Design review of the part shown in the three views and the two pictorial views. Dimensions are in mm from the part's minimum x, y and z. Give positions to 0.01 mm unless a question says otherwise; leave off trailing zeros. Loops run counter-clockwise (first coordinate to the right, second up) from the corner with the lowest first, then second, coordinate; pieces in that order, holes last. Notation, with made-up numbers: (64, 32) -> (93, 32) arc R20 ccw to (93, 54) -> close; hole circle Ø10 at (26, 57.25). An arc over 180 degrees is marked (long way). One line per question, with ' | ' between items. Start each with the question number.
(1) Insertion check: P1, Ø1.5, axis at y = 19.5, z = 27, coming from the -X side; P2, Ø1.5, axis at y = 17, z = 73, coming from the -X side; P3, Ø1.5, axis at x = 14.5, y = 15.5, coming from the +Z side. Each pin has a flat end and moves straight along its axis. Give the tip position at first contact, or say it passes through.
(2) Consider section C-C (z = 48.5). Write out the cut boundary in (x, y), and give its area (3 significant figures).
(3) Consider section A-A (y = 15). Write out the cut boundary in (x, z).
(4) Consider section B-B (z = 79). Write out the cut boundary in (x, y).
(5) Wall thickness on probe 1 along Y at (x, z) = (15, 71.25); probe 2 along X at (y, z) = (16, 72.5); probe 3 along X at (y, z) = (15.5, 73): over which ranges is each line inside the solid? List them lowest first.
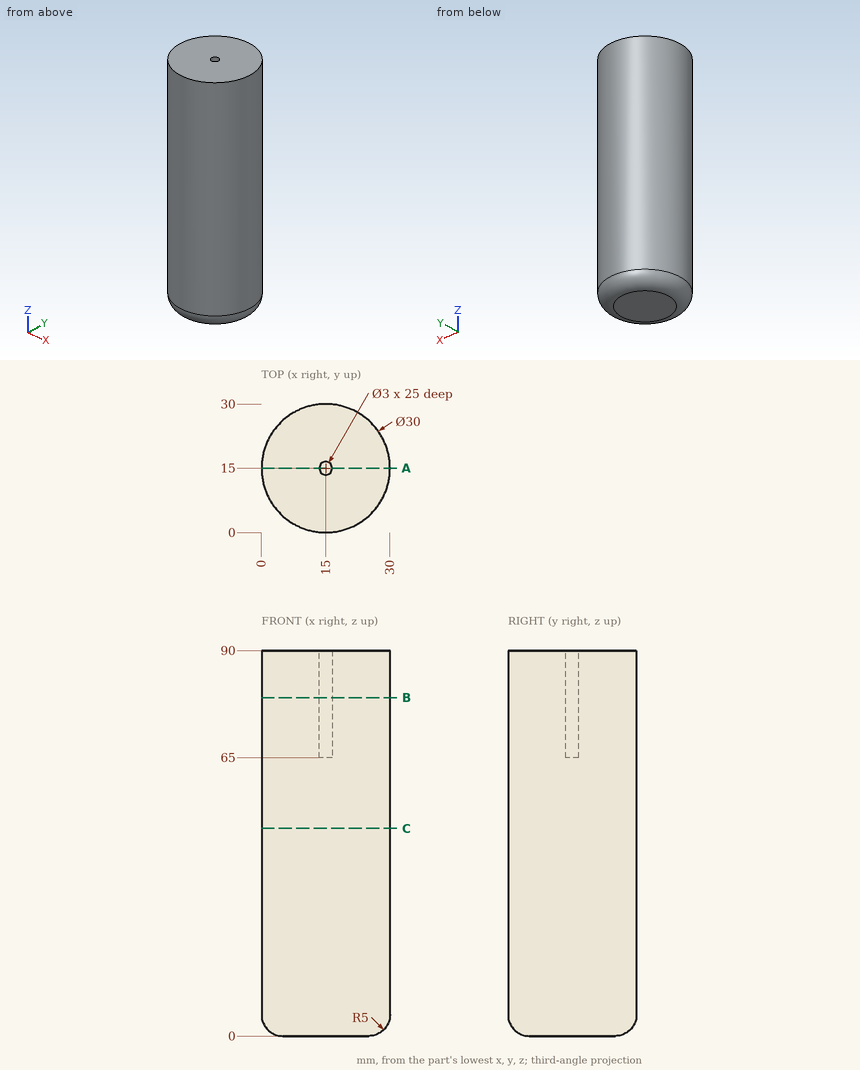
A:
1) P1: stops at x = 0.48 | P2: stops at x = 0.05 | P3: stops at z = 65
2) outline: circle Ø30 at (15, 15) | area: 707 mm^2
3) outline: (0, 5) arc R5 ccw to (5, 0) -> (25, 0) arc R5 ccw to (30, 5) -> (30, 90) -> (16.5, 90) -> (16.5, 65) -> (13.5, 65) -> (13.5, 90) -> (0, 90) -> close
4) outline: circle Ø30 at (15, 15); hole circle Ø3 at (15, 15)
5) probe 1: y = 0 to 13.5, 16.5 to 30 | probe 2: x = 0.03 to 13.88, 16.12 to 29.97 | probe 3: x = 0.01 to 13.59, 16.41 to 29.99
